Check sheet for the modelled part. Datum: model origin and axes. Units: mm. A direction names the side the tool comes from. Round coordinates to 2 decimals unless told otherwise and drop trailing zeros. Order: outer loops, then holes, each group sorted by start corner. A loop starts at its lowest first (then second) coordinate and runs counter-clockwise, first axis right, second up.
(1) Mould release check, pull along Y, two halves, no side actions. Record for faces 1 (the flat face through (-2.086, -3.546, 4.93)), 2 (the flat face through (-4.114, 0, 5)), 3 (the flat face through (-1.344, 2, 6)), 4 (the flat face through (1.344, -2, 6)): released by +Y, released by -Y, zero draft, split by the parting line, or undercut.
(2) Tool access check on faces 5 (the flat face through (2.086, 3.546, 4.93)), 6 (the flat face through (-2, -2, 4)), 7 (the flat face through (3.232, 0, 5)). Record the directions out of +Z, -Z, +X, -X, +Y, -Y that give a thin tool (end or side, any length) a straight path to the whole face; none if there is none.
(3) Depth check by flat-ended pin: pin 1 (2 mm diameter, centred on y = -2.5, z = 5, fed in from +X); pin 2 (0.9 mm diameter, centred on x = -2.5, z = 2.5, fed in from +Y); pin 3 (1.5 mm diameter, centred on x = 2.5, z = 3, fed in from +Y); pin 4 (3 mm diameter, centred on x = 0, z = 3.5, fed in from +Y). Enter the tip coordinate at first touch or a pass-through.
(4) Thickness scan on probe 1 along X at (y, z) = (2, 7); probe 2 along X at (y, z) = (-1, 3.75); probe 3 along Y at (x, z) = (-0.5, 9.25). Record the ranges inside material, lowest first.
(5) Sectioned sample at A-A, the plane y = 1. Enter the section's corners in (x, z), and give its area (3 significant figures).
(6) Sectioned sample at D-D, the plane y = -2. Enter the section's corners in (x, z), and give its area (3 significant figures).
(7) Sectioned sample at C-C, the plane x = -1. Enter the section's corners in (y, z).
```python
from build123d import *

# Parameters (mm, degrees)
PAD023_DEPTH    = 10
POCKET011_DEPTH = 10
SKETCH038_R     = 3
POCKET012_DEPTH = 4


with BuildPart() as part:
    # Sketch036 → Pad023 (new body)
    with BuildSketch(Plane.XY):
        Polygon((4.113621, -2.375), (4.113621, 2.375), (0, 4.75), (-4.113621, 2.375), (-4.113621, -2.375), (0, -4.75), align=None)
    extrude(amount=PAD023_DEPTH)

    # Sketch037 (on Face8 of Pad023) → Pocket011 (cut)
    with BuildSketch(Plane.XY.offset(10)):
        Polygon((-3.231873, -1.343503), (-3.231873, 1.343503), (-1.343503, 1.343503), (-1.343503, 3.231873), (1.343503, 3.231873), (1.343503, 1.343503), (3.231873, 1.343503), (3.231873, -1.343503), (1.343503, -1.343503), (1.343503, -3.231873), (-1.343503, -3.231873), (-1.343503, -1.343503), align=None)
    extrude(amount=-POCKET011_DEPTH, mode=Mode.SUBTRACT)

    # Sketch038 (on Face4 of Pocket011) → Pocket012 (cut)
    with BuildSketch(Plane(origin=(0, 0, 0), x_dir=(1, 0, 0), z_dir=(0, 0, -1))):
        Circle(SKETCH038_R)
    extrude(amount=-POCKET012_DEPTH, mode=Mode.SUBTRACT)


solid = part.part
```
Derived:
1. face 1: released by -Y
1. face 2: zero draft
1. face 3: undercut
1. face 4: undercut
2. face 5: +Z, -Z, +X, +Y
2. face 6: -Z
2. face 7: +Z, -Z
3. pin 1: stops at x = 4.11
3. pin 2: stops at y = 3.57
3. pin 3: stops at y = 3.74
3. pin 4: stops at y = 4.75
4. probe 1: x = -4.11 to -1.34, 1.34 to 4.11
4. probe 2: x = -4.11 to -3.23, 3.23 to 4.11
4. probe 3: y = -4.46 to -3.23, 3.23 to 4.46
5. outline: (-4.11, 0) - (-3.23, 0) - (-3.23, 10) - (-4.11, 10) - close; (3.23, 0) - (4.11, 0) - (4.11, 10) - (3.23, 10) - close
5. area: 17.6 mm2
6. outline: (-4.11, 0) - (-2.24, 0) - (-2.24, 4) - (-1.34, 4) - (-1.34, 10) - (-4.11, 10) - close; (1.34, 4) - (2.24, 4) - (2.24, 0) - (4.11, 0) - (4.11, 10) - (1.34, 10) - close
6. area: 48.3 mm2
7. outline: (-4.17, 0) - (-3.23, 0) - (-3.23, 10) - (-4.17, 10) - close; (3.23, 0) - (4.17, 0) - (4.17, 10) - (3.23, 10) - close
